Answer from the drawing. Dimensions are ordinates in mm from the lowest x, y and z of the part. Round coordinates to 2 decimals unless told otherwise and drop trailing zeros. Write each loop counter-clockwise with the first axis right and the second up, starting at its lowest first coordinate (ties: lowest second). Pieces come first, ordered by that corner, then holes. Notation, with made-up numbers: (72.5, 6) - (121.5, 6) arc R20 ccw to (121.5, 17) - close; hole circle Ø1 at (69, 16). An arc over 180 degrees is marked (long way). Return JSON: item names as keys, results as strings. Group by question number.
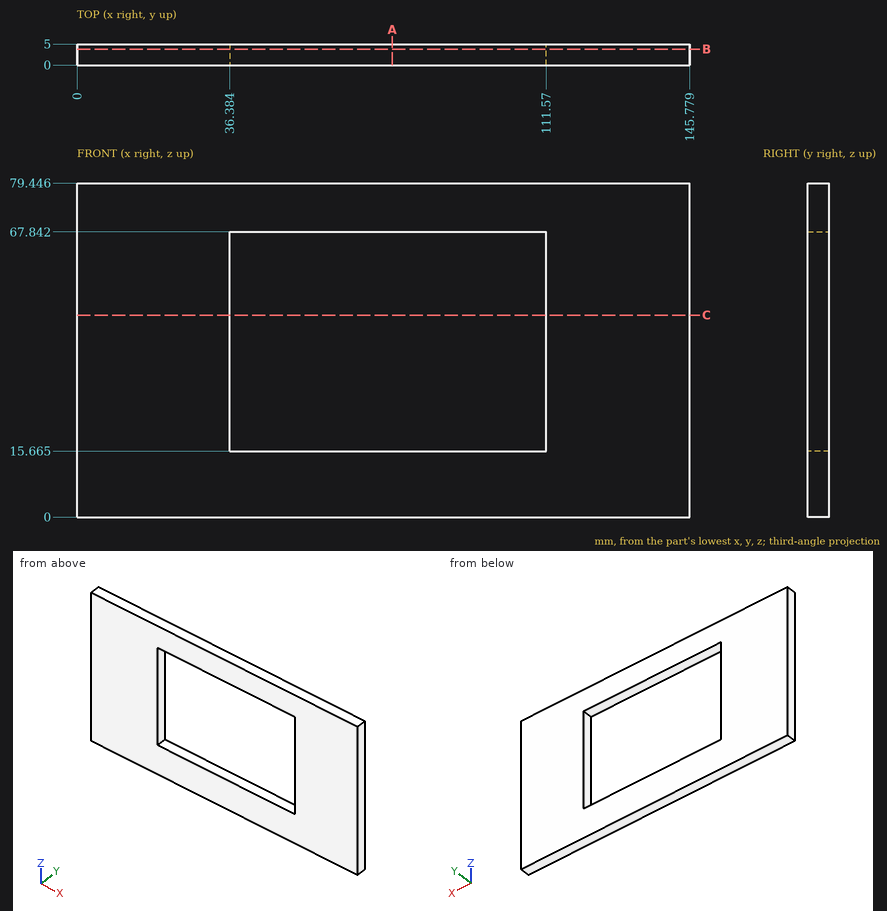
(1) Consider line 1 (X direction, y = 1.95, z = 54); line 2 (Z direction, x = 74.5, y = 3.7) (1 decimal). Determine where each line is inside the solid, lowest interval first.
(2) A flat-ended cylindrical pin translates along its axis: pin 1 (2 mm diameter, centred on x = 37, z = 49, fed in from -Y). Find the tip coordinate at first contact, or state that the pin passes through.
(3) Find section B-B (y = 3.8). Write down the section's boundary in (x, z) (1 decimal).
(4) Find section A-A (x = 75). Write down the section's boundary in (y, z) (1 decimal).
(5) Find section C-C (z = 48). Write down the section's boundary in (x, y), plus the area to 3 significant figures.
Check sheet entries:
{
 "1": {"line 1": "x = 0 to 36.38, 111.57 to 145.78", "line 2": "z = 0 to 15.7, 67.8 to 79.4"},
 "2": {"pin 1": "stops at y = 0"},
 "3": {"outline": "(0, 0) - (145.8, 0) - (145.8, 79.4) - (0, 79.4) - close; hole (36.4, 15.7) - (111.6, 15.7) - (111.6, 67.8) - (36.4, 67.8) - close"},
 "4": {"outline": "(0, 0) - (5, 0) - (5, 15.7) - (0, 15.7) - close; (0, 67.8) - (5, 67.8) - (5, 79.4) - (0, 79.4) - close"},
 "5": {"outline": "(0, 0) - (36.38, 0) - (36.38, 5) - (0, 5) - close; (111.57, 0) - (145.78, 0) - (145.78, 5) - (111.57, 5) - close", "area": "353 mm^2"}
}
